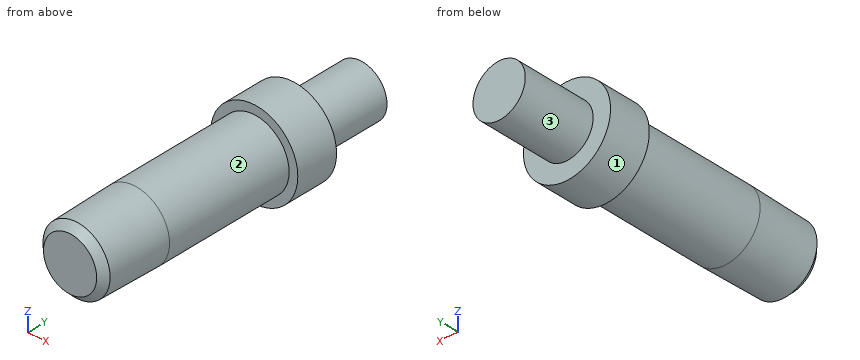
from build123d import *

# Parameters (mm, degrees)
SKETCH2_R           = 1.25
BOSS_EXTRUDE1_DEPTH = 9


with BuildPart() as part:
    # Sketch2 → Boss-Extrude1 (new body)
    with BuildSketch(Plane(origin=(0, 0, 0), x_dir=(1, 0, 0), z_dir=(0, 1, 0))):
        Circle(SKETCH2_R)
    extrude(amount=BOSS_EXTRUDE1_DEPTH)

    # Sketch4 → Cut-Revolve1 (revolve, cut)
    with BuildSketch(Plane.XY):
        Polygon((0.75, 9), (0.75, 6.9), (1.25, 6.9), (1.25, 5.7), (1, 5.7), (1, 2), (0.963866832, 0.2), (0.763866832, 0), (1.75, 0), (1.75, 9), align=None)
    revolve(axis=Axis((0, 9, 0), (0, -1, 0)), mode=Mode.SUBTRACT)


solid = part.part
Input: part model. Units: mm. Frame: model coordinates. Face numbers are marked on the shaded views. A direction names the side the tool comes from. Round coordinates to 2 decimals unless told otherwise and drop trailing zeros. Order: outer loops, then holes, each group sorted by start corner. A loop starts at its lowest first (then second) coordinate and runs counter-clockwise, first axis right, second up.
1. Cut plane B-B, the plane z = 0. Output: boundary loops of the cut face in (x, y), then the cut area to 3 significant figures.
The answers:
outline: (-1.25, 5.7) - (-1, 5.7) - (-1, 2) - (-0.96, 0.2) - (-0.76, 0) - (0.76, 0) - (0.96, 0.2) - (1, 2) - (1, 5.7) - (1.25, 5.7) - (1.25, 6.9) - (0.75, 6.9) - (0.75, 9) - (-0.75, 9) - (-0.75, 6.9) - (-1.25, 6.9) - close
area: 17.4 mm2
2. Set-up query: the marked faces 1, 2 and 3. Return all of +Z, -Z, +X, -X, +Y, -Y with unobstructed straight access to the full face (end or side cutting, diameter ignored); none if empty.
The answers:
face 1: +Y, -Y
face 2: -Y
face 3: +Y
3. Cut plane C-C, the plane y = 6. Output: boundary loops of the cut face in (x, z).
The answers:
outline: circle Ø2.5 at (0, 0)
4. Pin query (flat end, axial travel): P1, Ø1, axis at x = -1, y = 7.5, coming from the -Z side. Return the tip coordinate at first contact, or that it passes through.
The answers:
P1: stops at z = -0.56
5. Cut plane A-A, the plane x = 0. Output: boundary loops of the cut face in (y, z), then the cut area to 3 significant figures.
The answers:
outline: (0, -0.76) - (0.2, -0.96) - (2, -1) - (5.7, -1) - (5.7, -1.25) - (6.9, -1.25) - (6.9, -0.75) - (9, -0.75) - (9, 0.75) - (6.9, 0.75) - (6.9, 1.25) - (5.7, 1.25) - (5.7, 1) - (2, 1) - (0.2, 0.96) - (0, 0.76) - close
area: 17.4 mm2
6. Cut plane D-D, the plane y = 8.5. Output: boundary loops of the cut face in (x, z), then the cut area to 3 significant figures.
The answers:
outline: circle Ø1.5 at (0, 0)
area: 1.77 mm2
7. Material intervals for line 1 (Y direction, x = 1.1, z = -0.1); line 2 (Z direction, x = -0.2, y = 8.25); line 3 (X direction, y = 4.75, z = 0.7), sorted ascending.
The answers:
line 1: y = 5.7 to 6.9
line 2: z = -0.72 to 0.72
line 3: x = -0.71 to 0.71
